For this review, use the dimensioned drawing (mm, ordinates from the lowest corner) and the shaded views. A direction names the side the tool comes from. Coordinates: 2 decimals unless noted, no trailing zeros. Loops run counter-clockwise (first coordinate to the right, second up) from the corner with the lowest first, then second, coordinate; pieces in that order, holes last. Notation, with made-up numbers: (57.5, 47) - (112.5, 47) arc R7 ccw to (112.5, 60) - close; hole circle Ø7 at (12.5, 63). An arc over 180 degrees is marked (long way). Answer in a Markdown table with one row per item. Add a question column.
(1) We need section D-D on z = 3. Write out the cut boundary in (x, y).
(2) We need section A-A on y = 6.25. Write out the cut boundary in (x, z).
(3) For line 1 along Y through (x, z) = (5.25, 6.75); line 2 along X through (y, z) = (5.75, 1.75) (1 decimal); line 3 along Z through (x, y) = (11.75, 7.5) (1 decimal), list the stretches that pass through material, from the lowest coordinate up.
(4) For P1, Ø2, axis at x = 9.5, z = 9.5, coming from the -Y side; P2, Ø2.5, axis at x = 6, z = 6, coming from the -Y side, all flat-tipped, find the tip position at first contact; note any pin that passes through.
(5) Machinability: for the marked faces 4, 5, 6 and 7, which of the approach directions +Z, -Z, +X, -X, +Y, -Y give a long, thin tool a straight path to every point of the face, cutting with its end or side? Answer none if there is none.
(6) We need section C-C on x = 9.5. Write out the cut boundary in (y, z).
(7) We need section B-B on z = 7.75. Write out the cut boundary in (x, y).
(8) Mouldability with a two-part tool opening along X and no side actions: class the marked faces 1, 2 and 3 as +X half, -X half, draft (parallel to the pull), parting line (faces both ways), or undercut.
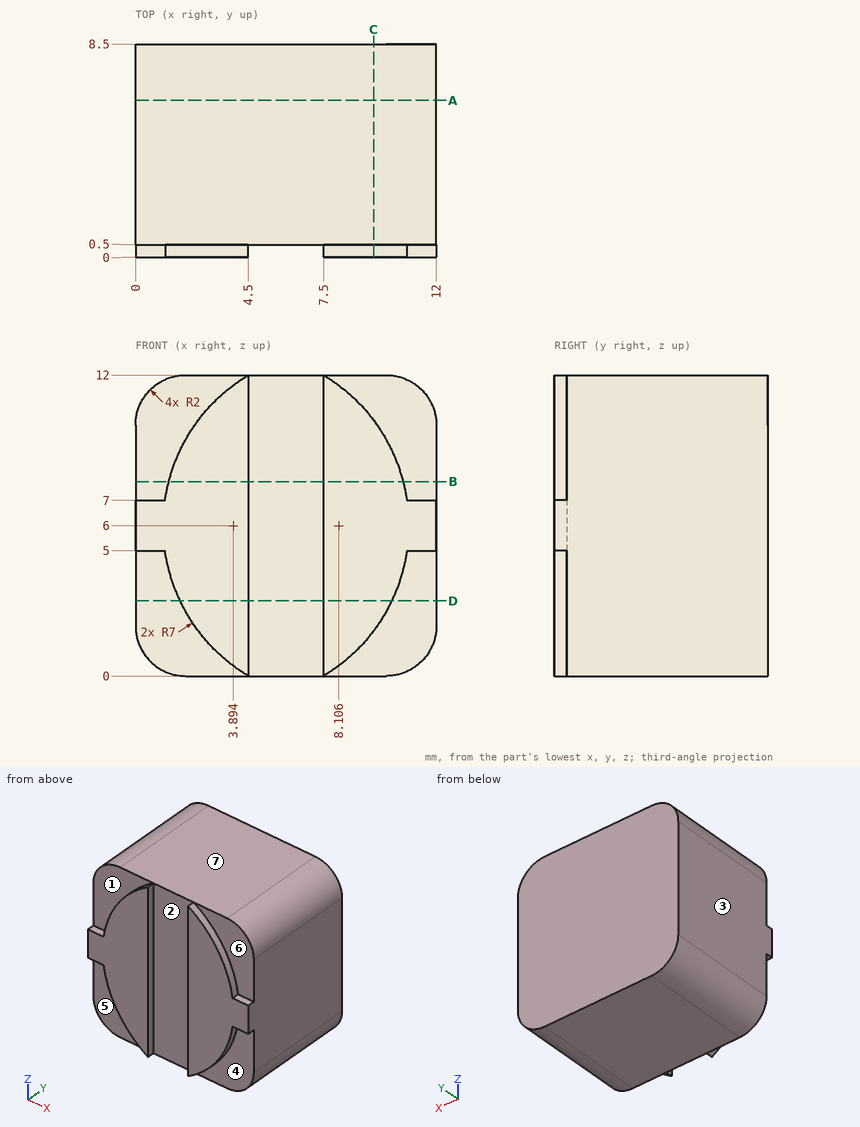
Outcome:
| question | item | result |
|---|---|---|
| 1 | outline | (0, 0.5) - (1.78, 0.5) - (1.78, 0) - (4.5, 0) - (4.5, 0.5) - (7.5, 0.5) - (7.5, 0) - (10.22, 0) - (10.22, 0.5) - (12, 0.5) - (12, 8.5) - (0, 8.5) - close |
| 2 | outline | (0, 2) arc R2 ccw to (2, 0) - (10, 0) arc R2 ccw to (12, 2) - (12, 10) arc R2 ccw to (10, 12) - (2, 12) arc R2 ccw to (0, 10) - close |
| 3 | line 1 | 0.5 to 8.5 |
| 3 | line 2 | 0 to 12 |
| 3 | line 3 | 1 to 11 |
| 4 | P1 | y = 0 |
| 4 | P2 | y = 0.5 |
| 5 | face 4 | -Z, +X, -Y |
| 5 | face 5 | -Z, -X, -Y |
| 5 | face 6 | +Z, +X, -Y |
| 5 | face 7 | +Z, +X, -X, +Y, -Y |
| 6 | outline | (0, 1.81) - (0.5, 1.81) - (0.5, 0) - (8.5, 0) - (8.5, 12) - (0.5, 12) - (0.5, 10.19) - (0, 10.19) - close |
| 7 | outline | (0, 0.5) - (1.33, 0.5) - (1.33, 0) - (4.5, 0) - (4.5, 0.5) - (7.5, 0.5) - (7.5, 0) - (10.67, 0) - (10.67, 0.5) - (12, 0.5) - (12, 8.5) - (0, 8.5) - close |
| 8 | face 1 | draft |
| 8 | face 2 | undercut |
| 8 | face 3 | -X half |
